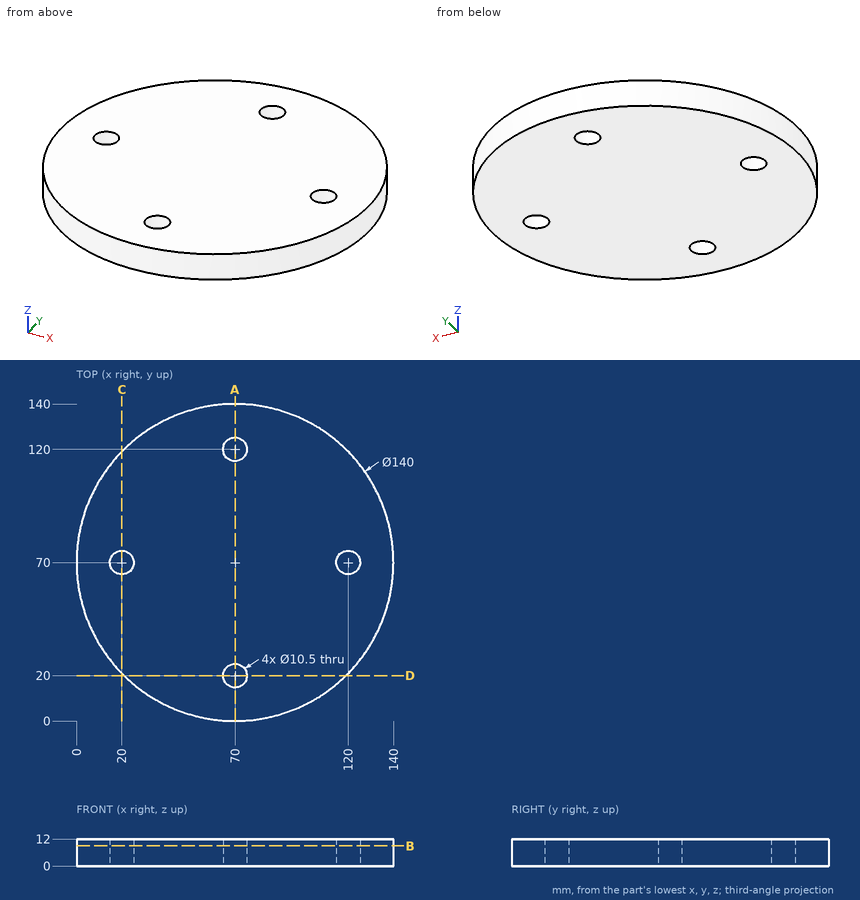
Geometry check sheet. Reference: drawing and pictorial views, mm from the part's lowest x, y, z. Round coordinates to 2 decimals unless told otherwise and drop trailing zeros. Order: outer loops, then holes, each group sorted by start corner. A loop starts at its lowest first (then second) coordinate and runs counter-clockwise, first axis right, second up. Notation, with made-up numbers: (72.5, 24) - (96.5, 24) arc R20 cw to (96.5, 29) - close; hole circle Ø3 at (65.25, 87). An arc over 180 degrees is marked (long way). One line per question, with ' | ' between items. Start each with the question number.
(1) Sectioned sample at A-A on x = 70. Record the cut outline in (y, z).
(2) Depth check by flat-ended pin: pin 1 Ø3 at (y, z) = (26.5, 6.5) entering from +X; pin 2 Ø1 at (x, z) = (96, 8.5) entering from +Y; pin 3 Ø3 at (x, z) = (88.5, 5.5) entering from +Y. Enter the tip coordinate at first touch or a pass-through.
(3) Sectioned sample at C-C on x = 20. Record the cut outline in (y, z).
(4) Sectioned sample at B-B on z = 9. Record the cut outline in (x, y), and give its area (3 significant figures).
(5) Thickness scan on L1, parallel to Y at x = 70, z = 2.75; L2, parallel to Y at x = 67, z = 2; L3, parallel to Y at x = 20, z = 6. Record the ranges inside material, lowest first. Write a range as [from, to].
Conclusion:
1) outline: (0, 0) - (14.75, 0) - (14.75, 12) - (0, 12) - close; (25.25, 0) - (114.75, 0) - (114.75, 12) - (25.25, 12) - close; (125.25, 0) - (140, 0) - (140, 12) - (125.25, 12) - close
2) pin 1: stops at x = 126 | pin 2: stops at y = 135.19 | pin 3: stops at y = 137.9
3) outline: (21.01, 0) - (64.75, 0) - (64.75, 12) - (21.01, 12) - close; (75.25, 0) - (118.99, 0) - (118.99, 12) - (75.25, 12) - close
4) outline: circle Ø140 at (70, 70); hole circle Ø10.5 at (20, 70); hole circle Ø10.5 at (70, 20); hole circle Ø10.5 at (70, 120); hole circle Ø10.5 at (120, 70) | area: 15,000 mm2
5) L1: y = [0, 14.75], [25.25, 114.75], [125.25, 140] | L2: y = [0.06, 15.69], [24.31, 115.69], [124.31, 139.94] | L3: y = [21.01, 64.75], [75.25, 118.99]
